The listing builds one solid part. Answer for the finished solid, in the listing's coordinates (mm). Round coordinates to 2 decimals unless told otherwise and drop trailing zeros. Loops run counter-clockwise (first coordinate to the right, second up) from the corner with the lowest first, then second, coordinate; pieces in that order, holes last. Notation, with made-up numbers: (-1, -13.5) -> (9, -13.5) arc R25 cw to (9, 12.5) -> close; hole circle Ø1 at (-15.5, -3). An arc over 180 degrees is marked (long way). One line per question, with ' | ' between items.
from build123d import *

# Parameters (mm, degrees)
F1_DEPTH = 40
F2_W     = 20
F2_H     = 3
F3_DEPTH = 25.4


with BuildPart() as f1:
    # F0 (on Top) → F1 (new body)
    with BuildSketch(Plane.XY):
        with BuildLine():
            ThreePointArc((0, 5.08), (1.487898, 1.487898), (5.08, 0))
            Line((5.08, 0), (124.92, 0))
            ThreePointArc((124.92, 0), (128.512102, 1.487898), (130, 5.08))
            Line((130, 5.08), (130, 47.92))
            ThreePointArc((130, 47.92), (128.512102, 51.512102), (124.92, 53))
            Line((124.92, 53), (5.08, 53))
            ThreePointArc((5.08, 53), (1.487898, 51.512102), (0, 47.92))
            Line((0, 47.92), (0, 5.08))
        make_face()
    extrude(amount=F1_DEPTH)

    # F2 (on face) → F3 (cut)
    with BuildSketch(Plane.XY.offset(40)):
        with Locations((15, 46.5)):
            Rectangle(F2_W, F2_H)
        with Locations((15, 38.5)):
            Rectangle(F2_W, F2_H)
        with Locations((15, 30.5)):
            Rectangle(F2_W, F2_H)
        with Locations((15, 22.5)):
            Rectangle(F2_W, F2_H)
        with Locations((15, 14.5)):
            Rectangle(F2_W, F2_H)
        with Locations((15, 6.5)):
            Rectangle(F2_W, F2_H)
        with Locations((40, 46.5)):
            Rectangle(F2_W, F2_H)
        with Locations((40, 38.5)):
            Rectangle(F2_W, F2_H)
        with Locations((40, 30.5)):
            Rectangle(F2_W, F2_H)
        with Locations((40, 22.5)):
            Rectangle(F2_W, F2_H)
        with Locations((40, 14.5)):
            Rectangle(F2_W, F2_H)
        with Locations((40, 6.5)):
            Rectangle(F2_W, F2_H)
        with Locations((65, 46.5)):
            Rectangle(F2_W, F2_H)
        with Locations((65, 38.5)):
            Rectangle(F2_W, F2_H)
        with Locations((65, 30.5)):
            Rectangle(F2_W, F2_H)
        with Locations((65, 22.5)):
            Rectangle(F2_W, F2_H)
        with Locations((65, 14.5)):
            Rectangle(F2_W, F2_H)
        with Locations((65, 6.5)):
            Rectangle(F2_W, F2_H)
        with Locations((90, 46.5)):
            Rectangle(F2_W, F2_H)
        with Locations((90, 38.5)):
            Rectangle(F2_W, F2_H)
        with Locations((90, 30.5)):
            Rectangle(F2_W, F2_H)
        with Locations((90, 22.5)):
            Rectangle(F2_W, F2_H)
        with Locations((90, 14.5)):
            Rectangle(F2_W, F2_H)
        with Locations((90, 6.5)):
            Rectangle(F2_W, F2_H)
        with Locations((115, 46.5)):
            Rectangle(F2_W, F2_H)
        with Locations((115, 38.5)):
            Rectangle(F2_W, F2_H)
        with Locations((115, 30.5)):
            Rectangle(F2_W, F2_H)
        with Locations((115, 22.5)):
            Rectangle(F2_W, F2_H)
        with Locations((115, 14.5)):
            Rectangle(F2_W, F2_H)
        with Locations((115, 6.5)):
            Rectangle(F2_W, F2_H)
    extrude(amount=-F3_DEPTH, mode=Mode.SUBTRACT)


solid = f1.part
Q1. A cutting plane is placed at B-B on z = 36.5. Give the number of separate pieces and of enclosed holes in the cut face, plus the area to 3 significant figures.
Numbers:
separate pieces: 1 | enclosed holes: 30 | area: 5,070 mm^2
Q2. A cutting plane is placed at A-A on x = 88. Give the vertices of the cut face in (y, z).
Numbers:
outline: (0, 0) -> (53, 0) -> (53, 40) -> (48, 40) -> (48, 14.6) -> (45, 14.6) -> (45, 40) -> (40, 40) -> (40, 14.6) -> (37, 14.6) -> (37, 40) -> (32, 40) -> (32, 14.6) -> (29, 14.6) -> (29, 40) -> (24, 40) -> (24, 14.6) -> (21, 14.6) -> (21, 40) -> (16, 40) -> (16, 14.6) -> (13, 14.6) -> (13, 40) -> (8, 40) -> (8, 14.6) -> (5, 14.6) -> (5, 40) -> (0, 40) -> close
Q3. Given pin 1 Ø0.9 at (x, y) = (14.5, 22.5) entering from +Z, flat-ended and moving along its own axis, determine where the tip first touches the part or whether it passes through.
Numbers:
pin 1: z = 14.6
Q4. For a pull along X with two mould halves and no side action, classify faces 1 (the face through (128.551, 51.472, 19.72)), 2 (the face through (64, 0, 20)), 3 (the face through (65, 13, 27)) as pulls with the +X half, pulls with the -X half, needs draft (parallel to the pull), parting line crosses it, or undercut.
Numbers:
face 1: pulls with the +X half | face 2: needs draft | face 3: undercut
Q5. Find the intervals of material crossed by line 1 (X direction, y = 37.5, z = 30); line 2 (Z direction, x = 44, y = 29.5); line 3 (X direction, y = 4, z = 25), in increasing order. Write a range as from..to.
Numbers:
line 1: 0..5, 25..30, 50..55, 75..80, 100..105, 125..130 | line 2: 0..14.6 | line 3: 0.12..129.88
